```python
from build123d import *

# Parameters (mm, degrees)
SKETCH1_W           = 22.5
SKETCH1_H           = 36
BOSS_EXTRUDE1_DEPTH = 1
SKETCH2_W           = 16.5
SKETCH2_H           = 16.5
BOSS_EXTRUDE2_DEPTH = 9.3
SKETCH3_R           = 7.5
BOSS_EXTRUDE3_DEPTH = 11
SKETCH4_R           = 7
BOSS_EXTRUDE4_DEPTH = 8.5
SKETCH5_W           = 9
SKETCH5_H           = 7.5
BOSS_EXTRUDE5_DEPTH = 3.5
SKETCH7_W           = 11
SKETCH7_H           = 15.6
BOSS_EXTRUDE6_DEPTH = 2


with BuildPart() as part:
    # Sketch1 → Boss-Extrude1 (new body)
    with BuildSketch(Plane.XY):
        Rectangle(SKETCH1_W, SKETCH1_H)
    extrude(amount=BOSS_EXTRUDE1_DEPTH)

    # Sketch2 → Boss-Extrude2 (add)
    with BuildSketch(Plane.XY.offset(1)):
        with Locations((0, 6.106677741)):
            Rectangle(SKETCH2_W, SKETCH2_H)
    extrude(amount=BOSS_EXTRUDE2_DEPTH)

    # Sketch3 → Boss-Extrude3 (add)
    with BuildSketch(Plane.XY.offset(10.3)):
        with Locations((0, 6.106677741)):
            Circle(SKETCH3_R)
    extrude(amount=BOSS_EXTRUDE3_DEPTH)

    # Sketch4 → Boss-Extrude4 (add)
    with BuildSketch(Plane.XY.offset(21.3)):
        with Locations((0, 6.106677741)):
            Circle(SKETCH4_R)
    extrude(amount=BOSS_EXTRUDE4_DEPTH)

    # Sketch5 → Boss-Extrude5 (add)
    with BuildSketch(Plane.XY.offset(1)):
        with Locations((0, -14.25)):
            Rectangle(SKETCH5_W, SKETCH5_H)
    extrude(amount=BOSS_EXTRUDE5_DEPTH)

    # Sketch7 → Boss-Extrude6 (add)
    with BuildSketch(Plane(origin=(0, 0, 0), x_dir=(-1, 0, 0), z_dir=(0, 0, -1))):
        with Locations((0, -10.2)):
            Rectangle(SKETCH7_W, SKETCH7_H)
    extrude(amount=BOSS_EXTRUDE6_DEPTH)


solid = part.part
```
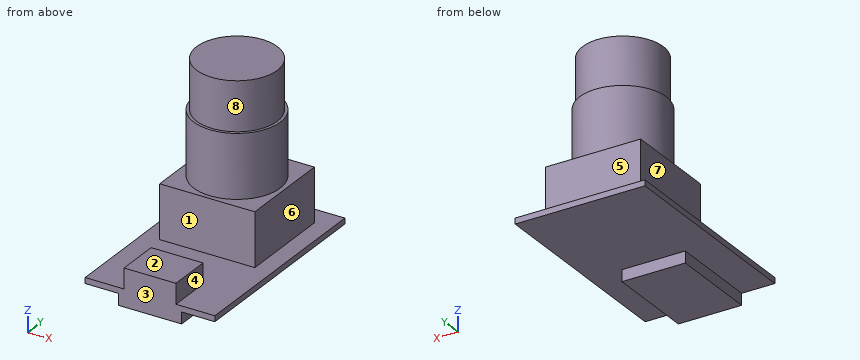
Check sheet for the modelled part. Datum: model origin and axes. Units: mm. Face numbers are marked on the shaded views. A direction names the side the tool comes from. Give positions to 0.01 mm unless a question says otherwise; leave off trailing zeros. Loops run counter-clockwise (first coordinate to the right, second up) from the corner with the lowest first, then second, coordinate; pieces in that order, holes last. Notation, with made-up numbers: M 59,-33 L 91,-33 A7 ccw 91,-29 Z; hole C 19.5,-11.75 d2. An arc over 180 degrees is marked long. Answer as CSV lines item,"result".
Item 1: Set-up check for the marked faces 4, 5, 6, 7 and 8: record each of +Z, -Z, +X, -X, +Y, -Y from which the full face is reachable in a straight line by a thin tool's end or side.
Reply:
face 4,"+Z, +X, -Y"
face 5,"+Z, +X, -X, +Y"
face 6,"+Z, +X, +Y, -Y"
face 7,"+Z, -X, +Y, -Y"
face 8,"+Z"
Item 2: Sectioned sample at C-C, the plane z = 7.5. Enter the section's corners in (x, y).
Reply:
outline,"M -8.25,-2.14 L 8.25,-2.14 L 8.25,14.36 L -8.25,14.36 Z"
Item 3: Scan lines: L1, parallel to Y at x = -3, z = 3; L2, parallel to Z at x = -1, y = 0; L3, parallel to Z at x = -7.5, y = 12.5. Record each from-to range of solid material in increasing order.
Reply:
L1,"-18 to -10.5, -2.14 to 14.36"
L2,"0 to 29.8"
L3,"0 to 10.3"
Item 4: Sectioned sample at B-B, the plane x = 0. Enter the section's corners in (y, z).
Reply:
outline,"M -18,-2 L -2.4,-2 L -2.4,0 L 18,0 L 18,1 L 14.36,1 L 14.36,10.3 L 13.61,10.3 L 13.61,21.3 L 13.11,21.3 L 13.11,29.8 L -0.89,29.8 L -0.89,21.3 L -1.39,21.3 L -1.39,10.3 L -2.14,10.3 L -2.14,1 L -10.5,1 L -10.5,4.5 L -18,4.5 Z"
Item 5: Sectioned sample at A-A, the plane y = -13. Enter the section's corners in (x, z), then the cut area to 3 significant figures.
Reply:
outline,"M -11.25,0 L -5.5,0 L -5.5,-2 L 5.5,-2 L 5.5,0 L 11.25,0 L 11.25,1 L 4.5,1 L 4.5,4.5 L -4.5,4.5 L -4.5,1 L -11.25,1 Z"
area,"76.0 mm^2"
Item 6: Sectioned sample at D-D, the plane y = 10. Enter the section's corners in (x, z).
Reply:
outline,"M -11.25,0 L 11.25,0 L 11.25,1 L 8.25,1 L 8.25,10.3 L 6.41,10.3 L 6.41,21.3 L 5.82,21.3 L 5.82,29.8 L -5.82,29.8 L -5.82,21.3 L -6.41,21.3 L -6.41,10.3 L -8.25,10.3 L -8.25,1 L -11.25,1 Z"
Item 7: Draft check along Y on the marked faces 1, 2 and 3. Enter one of: pulls with the +Y half, pulls with the -Y half, needs draft (parallel to the pull), parting line crosses it, or undercut.
Reply:
face 1,"undercut"
face 2,"needs draft"
face 3,"pulls with the -Y half"
Item 8: Depth check by flat-ended pin: pin 1 Ø3 at (y, z) = (8.5, 7.5) entering from -X; pin 2 Ø7.5 at (x, z) = (-3, 7.5) entering from +Y; pin 3 Ø10 at (y, z) = (-6, 11) entering from +X; pin 4 Ø1.6 at (y, z) = (-9, -0.5) entering from +X. Enter the tip coordinate at first touch or a pass-through.
Reply:
pin 1,"x = -8.25"
pin 2,"y = 14.36"
pin 3,"x = 8.25"
pin 4,"x = 11.25"
